Verification items for the finished model (mm, model axes). A direction names the side the tool comes from. Give positions to 0.01 mm unless a question says otherwise; leave off trailing zeros. Order: outer loops, then holes, each group sorted by start corner. A loop starts at its lowest first (then second) coordinate and runs counter-clockwise, first axis right, second up. Notation, with made-up numbers: M 5.5,39 L 37.5,39 A23 cw 37.5,54 Z; hole C 79.5,1 d4. An arc over 180 degrees is marked long. Answer as a JSON object with one key per item and string values.
Autodesk Inventor part; units mm, degrees
ref_plane "YZ Plane" through (0, 0, 0) normal (1, 0, 0) x (0, 1, 0)
ref_plane "XZ Plane" through (0, 0, 0) normal (0, 1, 0) x (-1, 0, 0)
ref_plane "XY Plane" through (0, 0, 0) normal (0, 0, 1) x (1, 0, 0)
sketch "Boceto1" plane through (0, 0, 0) normal (0, 0, 1) x (1, 0, 0)
  line L0 (-33.5, -15.5) -> (-33.5, 15.5)
  line L1 (-36.5, -15.5) -> (-33.5, -15.5)
  line L2 (-33.5, 15.5) -> (-36.5, 15.5)
  line L3 (-36.5, 15.5) -> (-36.5, -15.5)
  line L4 (36.5, -36.5) -> (36.5, 36.5)
  line L5 (-36.5, -36.5) -> (36.5, -36.5)
  line L6 (-36.5, 36.5) -> (-36.5, -36.5)
  line L7 (36.5, 36.5) -> (-36.5, 36.5)
  point P0 (0, 0)
extrude "Extrusión1" add sketch "Boceto1" along normal blind 3
sketch "Boceto2" plane through (0, 0, 3) normal (0, 0, 1) x (1, 0, 0)
  line L0 (36.5, 36.5) -> (-36.5, 36.5)
  line L1 (-36.5, 36.5) -> (-36.5, -36.5)
  line L2 (-36.5, -36.5) -> (36.5, -36.5)
  line L3 (36.5, -36.5) -> (36.5, 36.5)
  circle A0 centre (-31.4, 31.4) radius 2.1
  circle A1 centre (-31.4, -31.4) radius 2.1
  circle A2 centre (31.4, -31.4) radius 2.1
  circle A3 centre (31.4, 31.4) radius 2.1
  point P0 (0, 0)
hole "Agujero1" at (-31.4, 31.4, 3) at (-31.4, -31.4, 3) at (31.4, -31.4, 3) at (31.4, 31.4, 3) direction (0, 0, -1) diameter 3.2 depth 5
sketch "Boceto4" plane through (-36.5, -36.5, 0) normal (-1, 0, 0) x (0, 0, 1)
  line L0 (0, 73) -> (0, 0)
  line L1 (0, 0) -> (3, 0)
  line L2 (3, 73) -> (3, 0)
  line L3 (0, 73) -> (3, 73)
  line L4 (3, 73) -> (0, 73)
  line L5 (0, 73) -> (0, 65)
  line L6 (0, 65) -> (3, 65)
  line L7 (3, 65) -> (3, 73)
  point P0 (0, 36.5)
  dimension "d9" = 8
extrude "Extrusión2" add sketch "Boceto4" along normal blind 8 contours L3 L2 L6 L0
sketch "Boceto5" plane through (-44.5, -36.5, 0) normal (-1, 0, 0) x (0, 0, 1)
  line L0 (3, 65) -> (3, 73)
  line L1 (3, 73) -> (0, 73)
  line L2 (0, 73) -> (0, 65)
  line L3 (0, 65) -> (3, 65)
  line L4 (0, 73) -> (3, 65)
  circle A0 centre (1.5, 69) radius 6
  line L5 (0, 62) -> (3, 62)
  line L6 (3, 62) -> (3, 76)
  line L7 (3, 76) -> (0, 76)
  line L8 (0, 76) -> (0, 62)
  line L9 (0, 62) -> (3, 76) construction
  line L10 (3, 62) -> (0, 76) construction
  point P0 (0, 36.5)
  point P1 (3, 74.8095)
  point P2 (3, 63.1905)
  dimension "d12" = 12
extrude "Extrusión3" add sketch "Boceto5" along normal blind 3 contours L4 L1 L0 | L6 A0 L8 L3 | L3 L2 L4 | L1 L8 A0 L6 | L8 A0 L2
ref_plane "Plano de trabajo1" through (36.5, 0, 3) normal (0, 1, 0) x (1, 0, 0)
ref_plane "Plano de trabajo2" through (0, -36.5, 0) normal (-1, 0, 0) x (0, 0, 1)
mirror "Simetría1" about plane through (36.5, 0, 3) normal (0, 1, 0) of "Extrusión3", "Extrusión2"
mirror "Simetría2" about plane through (0, -36.5, 0) normal (-1, 0, 0) of "Extrusión3", "Extrusión2", "Simetría1"
sketch "Boceto6" plane through (36.5, -28.5, 0) normal (1, 0, 0) x (0, 0, -1)
  line L0 (0, 13) -> (75, 13)
  arc A0 (75, 7) -> (75, 13) centre (75, 10) ccw
  line L1 (75, 7) -> (0, 7)
  line L2 (0, -8) -> (0, 7)
  line L3 (81, -8) -> (0, -8)
  line L4 (81, -8) -> (81, 65)
  line L5 (81, 65) -> (0, 65)
  line L6 (0, 50) -> (0, 65)
  line L7 (0, 50) -> (75, 50)
  arc A1 (75, 44) -> (75, 50) centre (75, 47) ccw
  line L8 (75, 44) -> (0, 44)
  line L9 (0, 13) -> (0, 44)
  line L10 (0, 44) -> (0, 13)
  line L11 (-3, 0) -> (0, 0)
  line L12 (0, 0) -> (0, 57)
  line L13 (0, 57) -> (-3, 57)
  line L14 (-3, 0) -> (-3, 57)
  line L15 (3, 35.5) -> (-3, 35.5)
  line L16 (-3, 35.5) -> (-3, 20.5)
  line L17 (-3, 20.5) -> (3, 20.5)
  line L18 (3, 20.5) -> (3, 35.5)
  line L19 (3, 35.5) -> (-3, 20.5) construction
  line L20 (-3, 35.5) -> (3, 20.5) construction
  point P0 (0, 28.5)
  point P1 (0, 28)
  dimension "d15" = 6
  dimension "d16" = 15
extrude "Extrusión4" add sketch "Boceto6" along normal blind 3 contours L17 L14 L15 L9 | L9 L15 L18 L17
mirror "Simetría3" about plane through (0, -36.5, 0) normal (-1, 0, 0) of "Extrusión4"
properties part number "Tapa dispensador"
Q1. Section check A-A on x = -31.4. Record the cut outline in (y, z), then the cut area to 3 significant figures.
Resolved:
{"outline": "M -36.5,0 L -33,0 L -33,3 L -36.5,3 Z; M -29.8,0 L 29.8,0 L 29.8,3 L -29.8,3 Z; M 33,0 L 36.5,0 L 36.5,3 L 33,3 Z", "area": "200 mm²"}
Q2. Section check C-C on x = 40.5. Record the cut outline in (y, z).
Resolved:
{"outline": "M -36.5,0 L -28.5,0 L -28.5,3 L -36.5,3 Z; M 28.5,0 L 36.5,0 L 36.5,3 L 28.5,3 Z"}
Q3. Material ranges on L1, parallel to X at y = 31.4, z = 1.85; L2, parallel to Y at x = 31.4, z = 1.7; L3, parallel to Y at x = 41.5, z = 1.25, recorded low to high.
Resolved:
{"L1": "x = -47.5 to -33, -29.8 to 29.8, 33 to 47.5", "L2": "y = -36.5 to -33, -29.8 to 29.8, 33 to 36.5", "L3": "y = -36.5 to -28.5, 28.5 to 36.5"}
Q4. Section check D-D on y = 31.4. Record the cut outline in (x, z).
Resolved:
{"outline": "M -47.5,-4.4 L -44.5,-4.4 L -44.5,0 L -33,0 L -33,3 L -47.5,3 Z; M -29.8,0 L 29.8,0 L 29.8,3 L -29.8,3 Z; M 33,0 L 44.5,0 L 44.5,-4.4 L 47.5,-4.4 L 47.5,3 L 33,3 Z"}
Q5. Section check B-B on y = 6. Record the cut outline in (x, z).
Resolved:
{"outline": "M -39.5,-3 L -36.5,-3 L -36.5,0 L 36.5,0 L 36.5,-3 L 39.5,-3 L 39.5,3 L -39.5,3 Z"}
Q6. Gauge pin test, flat ends, axial feed: pin 1 Ø1.5 at (x, z) = (38.5, 1.5) entering from +Y; pin 2 Ø0.9 at (x, z) = (41.5, 1.5) entering from -Y; pin 3 Ø3 at (y, z) = (-3, -1.5) entering from -X; pin 4 Ø3.5 at (x, y) = (31.4, 31.4) entering from +Z. Record the tip position at first contact, or that the pin passes through.
Resolved:
{"pin 1": "stops at y = 36.5", "pin 2": "stops at y = -36.5", "pin 3": "stops at x = -39.5", "pin 4": "stops at z = 3"}
Q7. Tool access check on faces 1 (the face through (-1, -36.5, 1)), 2 (the face through (-40, -28.5, 2)), 3 (the face through (-36.5, 0, -2)). Record the directions out of +Z, -Z, +X, -X, +Y, -Y that give a thin tool (end or side, any length) a straight path to the whole face; none if there is none.
Resolved:
{"face 1": "+Z, -Z, -Y", "face 2": "+Z, -Z", "face 3": "-Z, +Y, -Y"}
Q8. Release check for a two-part mould opening along X. For faces 4 (the face through (40, -28.5, 1)), 5 (the face through (-30.43, 32.67, 1.48)), 6 (the face through (38, 7, 0)), 7 (the face through (39.5, 0, 0)) record: +X half, -X half, draft (parallel to the pull), parting line (faces both ways), or undercut.
Resolved:
{"face 4": "undercut", "face 5": "undercut", "face 6": "draft", "face 7": "+X half"}
